Verification items for the finished model (mm, model axes). Give positions to 0.01 mm unless a question says otherwise; leave off trailing zeros. Order: outer loops, then holes, each group sorted by start corner. A loop starts at its lowest first (then second) coordinate and runs counter-clockwise, first axis right, second up.
(1) Sectioned sample at D-D on x = 54.5. Record the cut outline in (y, z).
(2) Scan lines: L1, parallel to Y at x = -63.5, z = 32; L2, parallel to X at y = 16.5, z = 40.5; L3, parallel to X at y = 3.5, z = 24.5. Record each from-to range of solid material in increasing order.
(3) Sectioned sample at C-C on z = 30.5. Record the cut outline in (x, y), plus the area to 3 significant figures.
(4) Mould release check, pull along Y, two halves, no side actions. Record for faces 1 (the face through (-1.44, -74.39, 1.91)), 2 (the face through (-15.12, -11.59, 25.04)), 3 (the face through (23, 1, 0)): pulls with the +Y half, pulls with the -Y half, needs draft (parallel to the pull), parting line crosses it, or undercut.
(5) Sectioned sample at A-A on x = -63.5. Record the cut outline in (y, z), plus the area to 3 significant figures.
(6) Sectioned sample at B-B on y = 0. Record the cut outline in (x, z), plus the area to 3 significant figures.
```python
from build123d import *

# Parameters (mm, degrees)
F0_W     = 254
F0_H     = 152.4
F0_R     = 19.05
F1_DEPTH = 50.8
F2_R     = 6.35


with BuildPart() as f1:
    # F0 (on Top) → F1 (new body)
    with BuildSketch(Plane.XY):
        Rectangle(F0_W, F0_H)
        with Locations((-63.5, 0)):
            Circle(F0_R, mode=Mode.SUBTRACT)
        Circle(F0_R, mode=Mode.SUBTRACT)
        with Locations((63.5, 0)):
            Circle(F0_R, mode=Mode.SUBTRACT)
    extrude(amount=F1_DEPTH)

    # F2
    f2_edges = [f1.edges().sort_by_distance(p)[0] for p in [
        (0, -76.2, 50.8),
        (-127, 0, 50.8),
        (127, 0, 0),
        (127, 0, 50.8),
        (-127, -76.2, 25.4),
        (127, -76.2, 25.4),
        (0, -76.2, 0),
        (127, 76.2, 25.4),
        (-127, 76.2, 25.4),
        (0, 76.2, 0),
        (0, 76.2, 50.8),
    ]]
    fillet(f2_edges, radius=F2_R)


solid = f1.part
```
Ans:
1. outline: (-76.2, 6.35) arc R6.35 ccw to (-69.85, 0) - (-16.79, 0) - (-16.79, 50.8) - (-69.85, 50.8) arc R6.35 ccw to (-76.2, 44.45) - close; (16.79, 0) - (69.85, 0) arc R6.35 ccw to (76.2, 6.35) - (76.2, 44.45) arc R6.35 ccw to (69.85, 50.8) - (16.79, 50.8) - close
2. L1: y = -76.2 to -19.05, 19.05 to 76.2
2. L2: x = -127 to -73.02, -53.98 to -9.52, 9.52 to 53.98, 73.02 to 127
2. L3: x = -127 to -82.23, -44.77 to -18.73, 18.73 to 44.77, 82.23 to 127
3. outline: (-127, -69.85) arc R6.35 ccw to (-120.65, -76.2) - (120.65, -76.2) arc R6.35 ccw to (127, -69.85) - (127, 69.85) arc R6.35 ccw to (120.65, 76.2) - (-120.65, 76.2) arc R6.35 ccw to (-127, 69.85) - close; hole circle Ø38.1 at (-63.5, 0); hole circle Ø38.1 at (0, 0); hole circle Ø38.1 at (63.5, 0)
3. area: 35,300 mm2
4. face 1: pulls with the -Y half
4. face 2: undercut
4. face 3: needs draft
5. outline: (-76.2, 6.35) arc R6.35 ccw to (-69.85, 0) - (-19.05, 0) - (-19.05, 50.8) - (-69.85, 50.8) arc R6.35 ccw to (-76.2, 44.45) - close; (19.05, 0) - (69.85, 0) arc R6.35 ccw to (76.2, 6.35) - (76.2, 44.45) arc R6.35 ccw to (69.85, 50.8) - (19.05, 50.8) - close
5. area: 5,770 mm2
6. outline: (-127, 0) - (-82.55, 0) - (-82.55, 50.8) - (-120.65, 50.8) arc R6.35 ccw to (-127, 44.45) - close; (-44.45, 0) - (-19.05, 0) - (-19.05, 50.8) - (-44.45, 50.8) - close; (19.05, 0) - (44.45, 0) - (44.45, 50.8) - (19.05, 50.8) - close; (82.55, 0) - (120.65, 0) arc R6.35 ccw to (127, 6.35) - (127, 44.45) arc R6.35 ccw to (120.65, 50.8) - (82.55, 50.8) - close
6. area: 7,070 mm2
